from build123d import *

# Parameters (mm, degrees)
RACCORDO1_R                = 3
FORO_FILETTATO_M10_1_D     = 8.5
FORO_FILETTATO_M10_1_DEPTH = 27.5
FORO_FILETTATO_M10_1_TIP   = 2.553657631
RACCORDO2_R                = 10
RACCORDO3_R                = 4


with BuildPart() as part:
    # Schizzo1 → Rivoluzione1 (revolve)
    with BuildSketch(Plane(origin=(0, 0, 0), x_dir=(0, 0, -1), z_dir=(1, 0, 0)), mode=Mode.PRIVATE) as rivoluzione1_sk:
        Polygon((0, 0), (-45, 0), (-45, 5), (-42, 5), (-22.374431335, 48.236816584), (-2, 60), (0, 60), align=None)
    revolve(rivoluzione1_sk.sketch.rotate(Axis((0, 0, 0), (0, 1, 0)), 180), axis=Axis((0, 0, 0), (0, 1, 0)))

    # Raccordo1
    raccordo1_edges = [part.edges().sort_by_distance(p)[0] for p in [
        (0, 5, 42),
    ]]
    fillet(raccordo1_edges, radius=RACCORDO1_R)

    # Foro filettato M10-1
    with Locations(Plane.XZ):
        with Locations((0, 0)):
            Hole(FORO_FILETTATO_M10_1_D / 2, depth=FORO_FILETTATO_M10_1_DEPTH)
            with Locations((0, 0, -(FORO_FILETTATO_M10_1_DEPTH + FORO_FILETTATO_M10_1_TIP / 2))):  # 118° drill point
                Cone(0, FORO_FILETTATO_M10_1_D / 2, FORO_FILETTATO_M10_1_TIP, mode=Mode.SUBTRACT)

    # Raccordo2
    raccordo2_edges = [part.edges().sort_by_distance(p)[0] for p in [
        (0, 48.236816584, 22.374431335),
    ]]
    fillet(raccordo2_edges, radius=RACCORDO2_R)

    # Raccordo3
    raccordo3_edges = [part.edges().sort_by_distance(p)[0] for p in [
        (0, 60, 2),
    ]]
    fillet(raccordo3_edges, radius=RACCORDO3_R)


solid = part.part
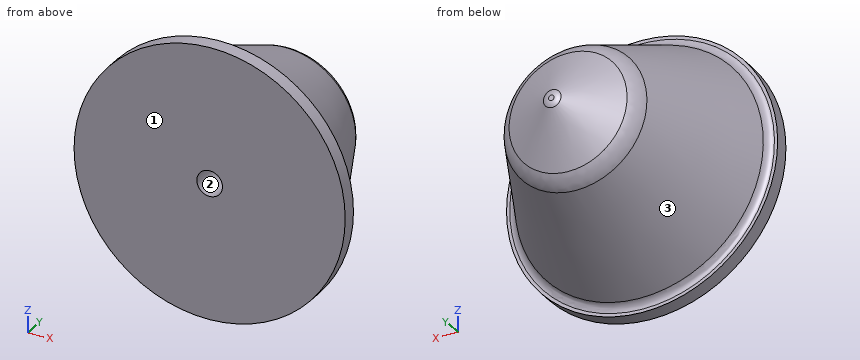
The model under review builds one solid part; all positions refer to its coordinate system, in mm. Face numbers are marked on the shaded views. Coordinates: 2 decimals unless noted, no trailing zeros. Order: outer loops, then holes, each group sorted by start corner. A loop starts at its lowest first (then second) coordinate and runs counter-clockwise, first axis right, second up. Notation, with made-up numbers: (27, 74.25) -> (43, 74.25) arc R12 cw to (43, 82.25) -> close; hole circle Ø3 at (9, 28.5). An arc over 180 degrees is marked (long way). Answer in a Markdown table with one row per item.
(1) Consider section A-A (y = 53.5). Write out the cut boundary in (x, z), plus the area to 3 significant figures.
Answers:
| item | result |
|---|---|
| outline | circle Ø26.52 at (0, 0) |
| area | 552 mm² |
(2) Consider section B-B (y = 36.5). Write out the cut boundary in (x, z), plus the area to 3 significant figures.
Answers:
| item | result |
|---|---|
| outline | circle Ø55.4 at (0, 0) |
| area | 2,410 mm² |
(3) Insertion check: pin 1 (2 mm diameter, centred on x = 0, y = 12.5, fed in from +Z); pin 2 (2 mm diameter, centred on x = -9.5, y = 34.5, fed in from -Z); pin 3 (8 mm diameter, centred on x = -28.5, z = -5.5, fed in from +Y); pin 4 (1.5 mm diameter, centred on x = -3.5, z = 2.5, fed in from -Y). Each pin has a flat end and moves straight along its axis. Give the tip position at first contact, or say it passes through.
Answers:
| item | result |
|---|---|
| pin 1 | z = 39.05 |
| pin 2 | z = -27.57 |
| pin 3 | y = 42.4 |
| pin 4 | y = 0 |
(4) Wall thickness on line 1 along Y through (x, z) = (16.5, 17); line 2 along X through (y, z) = (12, 0); line 3 along X through (y, z) = (15, 0): over which ranges is each line inside the solid? List them lowest first.
Answers:
| item | result |
|---|---|
| line 1 | 0 to 45.34 |
| line 2 | -38.82 to -4.25, 4.25 to 38.82 |
| line 3 | -37.46 to -4.25, 4.25 to 37.46 |
(5) The part is to be moulded in two halves that separate along Z. For the marked faces 1, 2 and 3, say which applies: +Z half, -Z half, draft (parallel to the pull), parting line (faces both ways), or undercut.
Answers:
| item | result |
|---|---|
| face 1 | draft |
| face 2 | undercut |
| face 3 | parting line |
